The listing builds one solid part. Answer for the finished solid, in the listing's coordinates (mm). A direction names the side the tool comes from. Coordinates: 2 decimals unless noted, no trailing zeros. Write each loop counter-clockwise with the first axis right and the second up, starting at its lowest first coordinate (ties: lowest second). Pieces come first, ordered by that corner, then holes.
```python
from build123d import *

# Parameters (mm, degrees)
SKETCH4_R          = 12.7
CUT_EXTRUDE1_DEPTH = 50.8


with BuildPart() as part:
    # Sketch2 → Revolve1 (revolve)
    with BuildSketch(Plane.XY):
        with BuildLine():
            Line((-11.947688608, 77.056557333), (-11.947688608, -170.628560352))
            Line((-11.947688608, -170.628560352), (-75.638147441, -170.628560352))
            Line((-75.638147441, -170.628560352), (-75.638147441, -18.228560352))
            add(Edge.make_bspline(
                [(-75.638147441, -18.228560352), (-41.40779095, 25.603897983), (-37.347688608, 77.056557333)],
                knots=[0, 0, 0, 1, 1, 1], degree=2))
            Line((-37.347688608, 77.056557333), (-11.947688608, 77.056557333))
        make_face()
    revolve(axis=Axis((-11.947688608, 77.056557333, 0), (0, -1, 0)))

    # Sketch3 → Revolve2 (revolve)
    with BuildSketch(Plane.XY, mode=Mode.PRIVATE) as revolve2_sk:
        with BuildLine():
            Line((-49.56693434, 48.997587312), (-41.94693434, 48.997587312))
            add(Edge.make_bspline(
                [(-37.347688606, 77.05655735), (-38.47805175, 62.73174853), (-41.946934336, 48.997587311)],
                knots=[0, 0, 0, 0.27840755, 0.27840755, 0.27840755], degree=2))
            Line((-37.347688606, 77.05655735), (-49.56693434, 77.05655735))
            Line((-49.56693434, 77.05655735), (-49.56693434, 48.997587312))
        make_face()
    revolve(revolve2_sk.sketch.rotate(Axis((-11.947688608, -170.628560352, 0), (0, 1, 0)), 180), axis=Axis((-11.947688608, -170.628560352, 0), (0, 1, 0)))

    # Sketch4 → Cut-Extrude1 (cut)
    with BuildSketch(Plane(origin=(0, 77.056557333, 0), x_dir=(1, 0, 0), z_dir=(0, 1, 0))):
        with Locations(Location((-11.947688608, 0, 0), (0, 0, 180))):
            Circle(SKETCH4_R)
    extrude(amount=-CUT_EXTRUDE1_DEPTH, mode=Mode.SUBTRACT)

    # Sketch5 → Cut-Revolve1 (revolve, cut)
    with BuildSketch(Plane.XY, mode=Mode.PRIVATE) as cut_revolve1_sk:
        with BuildLine():
            Line((-17.027688608, -165.548560352), (-17.027688608, 71.976557333))
            Line((-17.027688608, 71.976557333), (-32.715004421, 71.976557333))
            add(Edge.make_bspline(
                [(-32.715004421, 71.976557333), (-34.491548465, 55.152406634), (-38.639010582, 39.007317693), (-45.89970512, 21.587276989), (-46.742513348, 19.662046222), (-48.500048501, 15.832183135), (-49.416278966, 13.924686931), (-52.256576763, 8.26403653), (-54.274096029, 4.567347719), (-60.67628191, -6.3053686), (-65.409969255, -13.264423559), (-70.558147441, -19.965805759)],
                knots=[0, 0, 0, 0, 0.5, 0.5, 0.5625, 0.5625, 0.625, 0.625, 0.75, 0.75, 1, 1, 1, 1], degree=3))
            Line((-70.558147441, -19.965805759), (-70.558147441, -165.548560352))
            Line((-70.558147441, -165.548560352), (-17.027688608, -165.548560352))
        make_face()
    revolve(cut_revolve1_sk.sketch.rotate(Axis((-17.027688608, -165.548560352, 0), (0, 1, 0)), 180), axis=Axis((-17.027688608, -165.548560352, 0), (0, 1, 0)), mode=Mode.SUBTRACT)


solid = part.part
```
(1) Which of the six approach directions +Z, -Z, +X, -X, +Y, -Y give full straight-line access (tool end or side, diameter ignored) to faces 1 (the flat face through (-13, -170.629, -1)), 2 (the flat face through (-25, 71.977, 0))?
(2) Section A-A, the plane y = -22.5 is taken. Write down the section's boundary in (x, z).
(3) Find the intervals of material crossed by probe 1 along Y at (x, z) = (25, 6.5); probe 2 along Y at (x, z) = (-48, 9); probe 3 along Y at (x, z) = (-2.5, -5), in increasing order.
(4) Section B-B, the plane x = -44.5 is taken. State how many separate pieces and enclosed holes the cut face has, plus the area to 3 significant figures.
(5) Each of these flat-tipped pins is pushed along its axis until it touches: pin 1 (10 mm diameter, centred on x = 29, y = 6.5, fed in from +Z); pin 2 (1 mm diameter, centred on x = -8, y = 30, fed in from -Z); pin 3 (1 mm diameter, centred on x = 28.5, z = 38, fed in from +Y). Where does it stop, or does it pass through?
(6) For a pull along X with two mould halves and no side action, classify faces 3 (the cylindrical face through (5.411, 62.831, 33.375)), 4 (the cylindrical face through (0.74, 71.83, 0.56)), 5 (the flat face through (-28, 77.057, -1)) as pulls with the +X half, pulls with the -X half, needs draft (parallel to the pull), parting line crosses it, or undercut.
Solution:
1. face 1: +Z, -Z, +X, -X, -Y
1. face 2: none
2. outline: circle Ø127.38 at (-11.95, 0); hole circle Ø107.06 at (-17.03, 0)
3. probe 1: y = -170.63 to -165.55, -4.22 to 26.25, 49 to 77.06
3. probe 2: y = -170.63 to -165.55, 14.23 to 27.12, 49 to 77.06
3. probe 3: y = -170.63 to -165.55
4. separate pieces: 2
4. enclosed holes: 1
4. area: 5,540 mm2
5. pin 1: stops at z = 31.96
5. pin 2: stops at z = -36.01
5. pin 3: stops at y = -6.25
6. face 3: parting line crosses it
6. face 4: undercut
6. face 5: needs draft
